```python
from build123d import *

# Parameters (mm, degrees)
BOSS_EXTRUDE1_DEPTH = 4
FILLET1_R           = 20
SKETCH1_R           = 2.25
SKETCH1_R_2         = 2.75
CUT_EXTRUDE3_DEPTH  = 131.855321132
BOSS_EXTRUDE2_START = 20
BOSS_EXTRUDE2_DEPTH = 20
SKETCH7_W           = 10
SKETCH7_H           = 20
BOSS_EXTRUDE3_DEPTH = 20
SKETCH8_W           = 12.2
SKETCH8_H           = 12.2
CUT_EXTRUDE4_DEPTH  = 3.1
CUT_EXTRUDE5_REACH  = 88.267
SKETCH8_3_W         = 12.2
SKETCH8_3_H         = 3.5


with BuildPart() as part:
    # Sketch3 → Boss-Extrude1 (new body)
    with BuildSketch(Plane(origin=(0, 0, 0), x_dir=(1, 0, 0), z_dir=(0, 1, 0))):
        with BuildLine():
            Line((22.912878475, 10), (44, 10))
            Line((44, 10), (44, 25))
            Line((44, 25), (54, 25))
            Line((54, 25), (54, -10))
            Line((54, -10), (22.912878475, -10))
            ThreePointArc((22.912878475, -10), (-25, 0), (22.912878475, 10))
        make_face()
    extrude(amount=BOSS_EXTRUDE1_DEPTH)

    # Fillet1
    fillet1_edges = [part.edges().sort_by_distance(p)[0] for p in [
        (22.912878475, 2, 10),
        (22.912878475, 2, -10),
    ]]
    fillet(fillet1_edges, radius=FILLET1_R)

    # Sketch1 → Cut-Extrude3 (cut, through all)
    with BuildSketch(Plane(origin=(103.38268991, 0, 0), x_dir=(1, 0, 0), z_dir=(0, 1, 0))):
        with Locations(Location((-103.38268991, 14.5, 0), (0, 0, 270))):
            Circle(SKETCH1_R)
        with Locations(Location((-103.38268991, -14.5, 0), (0, 0, 270))):
            Circle(SKETCH1_R)
        with Locations(Location((-66.469811435, 0, 0), (0, 0, 270))):
            Circle(SKETCH1_R_2)
    extrude(amount=CUT_EXTRUDE3_DEPTH, mode=Mode.SUBTRACT)

    # Sketch4 → Boss-Extrude2 (add)
    with BuildSketch(Plane.XZ.offset(BOSS_EXTRUDE2_START)):
        with BuildLine():
            Line((18.633899812, 16.666666667), (17.452315988, 15.609825965))
            ThreePointArc((17.452315988, 15.609825965), (16.092851842, 15.100708662), (14.747154343, 15.645173018))
            ThreePointArc((14.747154343, 15.645173018), (-21.5, 0), (14.747154343, -15.645173018))
            ThreePointArc((14.747154343, -15.645173018), (16.092851842, -15.100708662), (17.452315988, -15.609825965))
            Line((17.452315988, -15.609825965), (18.633899812, -16.666666667))
            ThreePointArc((18.633899812, -16.666666667), (-25, 0), (18.633899812, 16.666666667))
        make_face()
    extrude(amount=-BOSS_EXTRUDE2_DEPTH)

    # Sketch7 → Boss-Extrude3 (add)
    with BuildSketch(Plane(origin=(0, 4, 0), x_dir=(1, 0, 0), z_dir=(0, 1, 0))):
        with Locations((49, 15)):
            Rectangle(SKETCH7_W, SKETCH7_H)
    extrude(amount=BOSS_EXTRUDE3_DEPTH)

    # Sketch8 → Cut-Extrude4 (cut)
    with BuildSketch(Plane(origin=(54, 0, 0), x_dir=(0, 0, -1), z_dir=(1, 0, 0))):
        with Locations((15, 12)):
            Rectangle(SKETCH8_W, SKETCH8_H)
    extrude(amount=-CUT_EXTRUDE4_DEPTH, mode=Mode.SUBTRACT)

    # Sketch8_3 → Cut-Extrude5 (cut, up to next)
    with BuildSketch(Plane(origin=(54, 0, 0), x_dir=(0, 0, -1), z_dir=(1, 0, 0)), mode=Mode.PRIVATE) as cut_extrude5_sk1:
        with Locations((15, 18.1)):
            Rectangle(SKETCH8_3_W, SKETCH8_3_H)
    cut_extrude5_tool1 = extrude(cut_extrude5_sk1.sketch, amount=-CUT_EXTRUDE5_REACH, mode=Mode.PRIVATE) & part.part
    add(cut_extrude5_tool1.solids().sort_by_distance((54, 18.1, -15))[0], mode=Mode.SUBTRACT)


solid = part.part
```
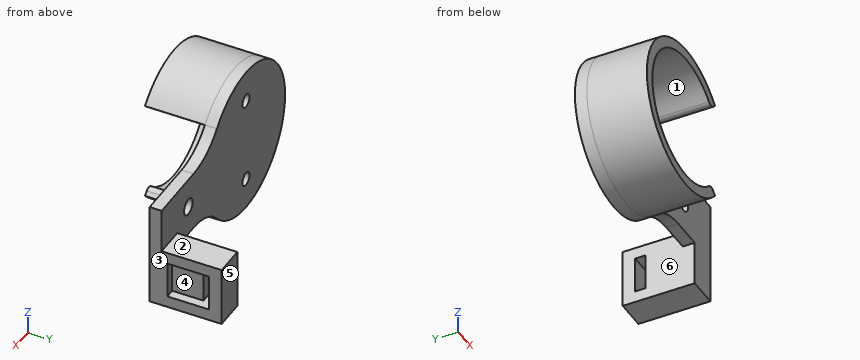
Verification items for the finished model (mm, model axes). Face numbers are marked on the shaded views. A direction names the side the tool comes from. Coordinates: 2 decimals unless noted, no trailing zeros. Order: outer loops, then holes, each group sorted by start corner. A loop starts at its lowest first (then second) coordinate and runs counter-clockwise, first axis right, second up. Notation, with made-up numbers: (81.5, 23) -> (121.5, 23) arc R24 cw to (121.5, 40) -> close; hole circle Ø9 at (66, 73). An arc over 180 degrees is marked (long way). Answer as CSV lines item,"result". Start each with the question number.
1) Material ranges on L1, parallel to Z at x = 0, y = 1.3; L2, parallel to X at y = 2, z = -14; L3, parallel to X at y = 1.95, z = -14.5, recorded low to high. Write a range as [from, to].
2) Cross-section at A-A, the plane x = 0. Record the boundary of the cut face in (y, z).
3) Release check for a two-part mould opening along Y. For the marked faces 4, 5 and 6 record: released by +Y, released by -Y, zero draft, split by the parting line, or undercut.
4) Set-up check for the marked faces 1, 2 and 3: record each of +Z, -Z, +X, -X, +Y, -Y from which the full face is reachable in a straight line by a thin tool's end or side.
5) Cross-section at D-D, the plane y = 13.5. Record the boundary of the cut face in (x, z).
6) Cross-section at B-B, the plane z = 0. Record the boundary of the cut face in (x, y).
7) Cross-section at C-C, the plane y = 19. Record the boundary of the cut face in (x, z).
8) Gauge pin test, flat ends, axial feed: pin 1 Ø14 at (x, z) = (30, -9.5) entering from -Y; pin 2 Ø8 at (y, z) = (-5.5, 10) entering from -X; pin 3 Ø11 at (x, y) = (48.5, 14) entering from +Z; pin 4 Ø4.5 at (x, z) = (36.91, 0) entering from +Y. Record the tip position at first contact, or that the pin passes through.
Conclusion:
1,L1,"z = [-25, -16.75], [-12.25, 12.25], [16.75, 25]"
1,L2,"x = [-20.71, -2.19], [2.19, 21.54], [44, 54]"
1,L3,"x = [-20.37, -2.25], [2.25, 20.9], [44, 54]"
2,outline,"(-20, -25) -> (4, -25) -> (4, -16.75) -> (0, -16.75) -> (0, -21.5) -> (-20, -21.5) -> close; (-20, 21.5) -> (0, 21.5) -> (0, 16.75) -> (4, 16.75) -> (4, 25) -> (-20, 25) -> close; (0, -12.25) -> (4, -12.25) -> (4, 12.25) -> (0, 12.25) -> close"
3,face 4,"undercut"
3,face 5,"released by +Y"
3,face 6,"zero draft"
4,face 1,"-Y"
4,face 2,"+Z, +X, -X, +Y"
4,face 3,"+Z, -Z, +X, +Y, -Y"
5,outline,"(44, -25) -> (54, -25) -> (54, -21.1) -> (50.9, -21.1) -> (50.9, -8.9) -> (54, -8.9) -> (54, -5) -> (44, -5) -> close"
6,outline,"(-25, -20) -> (-21.5, -20) -> (-21.5, 0) -> (34.16, 0) -> (34.16, 4) -> (-25, 4) -> close; (39.66, 0) -> (54, 0) -> (54, 4) -> (39.66, 4) -> close"
7,outline,"(44, -25) -> (54, -25) -> (54, -21.1) -> (44, -21.1) -> close; (44, -8.9) -> (54, -8.9) -> (54, -5) -> (44, -5) -> close"
8,pin 1,"stops at y = 0"
8,pin 2,"stops at x = -24.27"
8,pin 3,"stops at z = -5"
8,pin 4,"passes through"
